Source: CAD feature listing. Evaluate the final solid. Frame: model axes, mm. A direction names the side the tool comes from. Coordinates: 2 decimals unless noted, no trailing zeros. Write each loop counter-clockwise with the first axis right and the second up, starting at its lowest first coordinate (ties: lowest second). Pieces come first, ordered by that corner, then holes. Notation, with made-up numbers: (-9.75, -9.5) - (30.25, -9.5) arc R21 ccw to (30.25, 24.5) - close; hole circle Ø1 at (-31.5, 9). An arc over 180 degrees is marked (long way). One line per item, written item: value.
from build123d import *

# Parameters (mm, degrees)
BOSS_EXTRUDE1_DEPTH       = 31
SKETCH2_W                 = 4
SKETCH2_H                 = 6
CUT_EXTRUDE1_DEPTH        = 10
CHAMFER1_SIZE             = 3
SKETCH3_R                 = 1
CUT_EXTRUDE2_DEPTH        = 12
SKETCH4_R                 = 2.75
CUT_EXTRUDE3_DEPTH        = 3
M3X0_5_TAPPED_HOLE1_D     = 2.5
M3X0_5_TAPPED_HOLE1_DEPTH = 5.5
M3X0_5_TAPPED_HOLE1_TIP   = 0.751075774
CHAMFER2_SIZE             = 1
CHAMFER3_SIZE             = 1
CHAMFER4_SIZE             = 1
CHAMFER5_SIZE             = 1
CHAMFER6_SIZE             = 1
SKETCH6_R                 = 3
CUT_EXTRUDE4_DEPTH        = 76.325976363
SKETCH7_R                 = 8.5
CUT_EXTRUDE5_DEPTH        = 8
CHAMFER7_SIZE             = 0.5
CHAMFER8_SIZE             = 0.5
SKETCH8_R                 = 3.25
CUT_EXTRUDE6_DEPTH        = 73.401676189
SKETCH9_R                 = 1
CUT_EXTRUDE7_DEPTH        = 26
CIRPATTERN1_COUNT         = 4


with BuildPart() as part:
    # Sketch1 → Boss-Extrude1 (new body)
    with BuildSketch(Plane(origin=(0, 0, 0), x_dir=(1, 0, 0), z_dir=(0, 1, 0))):
        with BuildLine():
            Line((38.438211647, 10.935520299), (38.438211647, 20.93675572))
            Line((38.438211647, 20.93675572), (42.438211647, 20.93675572))
            Line((42.438211647, 20.93675572), (42.438211647, 14.546924278))
            ThreePointArc((42.438211647, 14.546924278), (61.123879761, -10.180568437), (38.22154498, -31.06324428))
            Line((38.22154498, -31.06324428), (-18.77845502, -31.06324428))
            Line((-18.77845502, -31.06324428), (-18.77845502, 14.93675572))
            Line((-18.77845502, 14.93675572), (33.82154498, 14.93675572))
            Line((33.82154498, 14.93675572), (33.82154498, 20.93675572))
            Line((33.82154498, 20.93675572), (37.82154498, 20.93675572))
            Line((37.82154498, 20.93675572), (37.82154498, 10.932544727))
            ThreePointArc((37.82154498, 10.932544727), (38.31322372, -27.063023095), (38.438211647, 10.935520299))
        make_face()
        with BuildLine():
            Line((12, 11.93675572), (12, 1.788697084))
            Line((12, 1.788697084), (16.336864234, 1.788697084))
            ThreePointArc((16.336864234, 1.788697084), (19.928181819, 7.472291251), (24.955045819, 11.93675572))
            Line((24.955045819, 11.93675572), (12, 11.93675572))
        make_face(mode=Mode.SUBTRACT)
        with BuildLine():
            Line((12, -17.915185645), (16.336864234, -17.915185645))
            ThreePointArc((16.336864234, -17.915185645), (19.928181819, -23.598779812), (24.955045819, -28.06324428))
            Line((24.955045819, -28.06324428), (12, -28.06324428))
            Line((12, -28.06324428), (12, -17.915185645))
        make_face(mode=Mode.SUBTRACT)
    extrude(amount=BOSS_EXTRUDE1_DEPTH)

    # Sketch2 → Cut-Extrude1 (cut)
    with BuildSketch(Plane(origin=(0, 31, 0), x_dir=(1, 0, 0), z_dir=(0, 1, 0))):
        with BuildLine():
            Line((38.438211647, 20.93675572), (38.438211647, 14.93675572))
            ThreePointArc((38.438211647, 14.93675572), (40.446719395, 14.829888823), (42.438211647, 14.547962381))
            Line((42.438211647, 14.547962381), (42.438211647, 20.93675572))
            Line((42.438211647, 20.93675572), (38.438211647, 20.93675572))
        make_face()
        with Locations((35.82154498, 17.93675572)):
            Rectangle(SKETCH2_W, SKETCH2_H)
    cut_extrude1 = extrude(amount=-CUT_EXTRUDE1_DEPTH, mode=Mode.SUBTRACT)

    # Mirror1: Cut-Extrude1 across plane
    add(cut_extrude1.mirror(Plane.ZX.offset(15.5)), mode=Mode.SUBTRACT)

    # Chamfer1
    chamfer1_edges = [part.edges().sort_by_distance(p)[0] for p in [
        (40.438211647, 10, -20.93675572),
        (35.82154498, 10, -20.93675572),
        (40.438211647, 21, -20.93675572),
        (35.82154498, 21, -20.93675572),
    ]]
    chamfer(chamfer1_edges, length=CHAMFER1_SIZE)

    # Sketch3 → Cut-Extrude2 (cut)
    with BuildSketch(Plane(origin=(42.438211647, 0, 0), x_dir=(0, 0, -1), z_dir=(1, 0, 0))):
        with Locations((17.73675572, 15.5)):
            Circle(SKETCH3_R)
    extrude(amount=-CUT_EXTRUDE2_DEPTH, mode=Mode.SUBTRACT)

    # Sketch4 → Cut-Extrude3 (cut)
    with BuildSketch(Plane(origin=(42.438211647, 0, 0), x_dir=(0, 0, -1), z_dir=(1, 0, 0))):
        with Locations((17.73675572, 15.5)):
            Circle(SKETCH4_R)
    extrude(amount=-CUT_EXTRUDE3_DEPTH, mode=Mode.SUBTRACT)

    # M3x0.5 Tapped Hole1
    with Locations(Plane(origin=(33.82154498, 15.5, -17.73675572), x_dir=(0, 0, -1), z_dir=(-1, 0, 0))):
        with Locations((0, 0)):
            Hole(M3X0_5_TAPPED_HOLE1_D / 2, depth=M3X0_5_TAPPED_HOLE1_DEPTH)
            with Locations((0, 0, -(M3X0_5_TAPPED_HOLE1_DEPTH + M3X0_5_TAPPED_HOLE1_TIP / 2))):  # 118° drill point
                Cone(0, M3X0_5_TAPPED_HOLE1_D / 2, M3X0_5_TAPPED_HOLE1_TIP, mode=Mode.SUBTRACT)

    # Chamfer2
    chamfer2_edges = [part.edges().sort_by_distance(p)[0] for p in [
        (61.123879761, 31, 10.180568437),
        (9.52154498, 31, -14.93675572),
        (-18.77845502, 31, 8.06324428),
        (9.72154498, 31, 31.06324428),
    ]]
    chamfer(chamfer2_edges, length=CHAMFER2_SIZE)

    # Chamfer3
    chamfer3_edges = [part.edges().sort_by_distance(p)[0] for p in [
        (40.446719395, 31, -14.829888823),
    ]]
    chamfer(chamfer3_edges, length=CHAMFER3_SIZE)

    # Chamfer4
    chamfer4_edges = [part.edges().sort_by_distance(p)[0] for p in [
        (9.52154498, 0, -14.93675572),
        (61.123879761, 0, 10.180568437),
        (9.72154498, 0, 31.06324428),
        (-18.77845502, 0, 8.06324428),
    ]]
    chamfer(chamfer4_edges, length=CHAMFER4_SIZE)

    # Chamfer5
    chamfer5_edges = [part.edges().sort_by_distance(p)[0] for p in [
        (40.446719395, 0, -14.829888823),
    ]]
    chamfer(chamfer5_edges, length=CHAMFER5_SIZE)

    # Chamfer6
    chamfer6_edges = [part.edges().sort_by_distance(p)[0] for p in [
        (-18.77845502, 15.5, -14.93675572),
        (-18.77845502, 15.5, 31.06324428),
    ]]
    chamfer(chamfer6_edges, length=CHAMFER6_SIZE)

    # Sketch6 → Cut-Extrude4 (cut, through all)
    with BuildSketch(Plane(origin=(0, 31, 0), x_dir=(1, 0, 0), z_dir=(0, 1, 0))):
        with Locations(Location((-5.77845502, -24.06324428, 0), (0, 0, 270))):
            Circle(SKETCH6_R)
        with Locations(Location((-5.77845502, 7.93675572, 0), (0, 0, 270))):
            Circle(SKETCH6_R)
    extrude(amount=-CUT_EXTRUDE4_DEPTH, mode=Mode.SUBTRACT)

    # Sketch7 → Cut-Extrude5 (cut)
    with BuildSketch(Plane(origin=(0, 31, 0), x_dir=(1, 0, 0), z_dir=(0, 1, 0))):
        with Locations(Location((-5.77845502, -8.06324428, 0), (0, 0, 270))):
            Circle(SKETCH7_R)
    cut_extrude5 = extrude(amount=-CUT_EXTRUDE5_DEPTH, mode=Mode.SUBTRACT)

    # Chamfer7
    chamfer7_edges = [part.edges().sort_by_distance(p)[0] for p in [
        (-5.77845502, 31, -0.43675572),
    ]]
    chamfer(chamfer7_edges, length=CHAMFER7_SIZE)

    # Mirror3: Cut-Extrude5 across plane
    add(cut_extrude5.mirror(Plane.ZX.offset(15.5)), mode=Mode.SUBTRACT)

    # Chamfer8
    chamfer8_edges = [part.edges().sort_by_distance(p)[0] for p in [
        (-5.77845502, 0, -0.43675572),
    ]]
    chamfer(chamfer8_edges, length=CHAMFER8_SIZE)

    # Sketch8 → Cut-Extrude6 (cut, through all)
    with BuildSketch(Plane(origin=(0, 23, 0), x_dir=(1, 0, 0), z_dir=(0, 1, 0))):
        with Locations(Location((-5.77845502, -8.06324428, 0), (0, 0, 270))):
            Circle(SKETCH8_R)
    extrude(amount=-CUT_EXTRUDE6_DEPTH, mode=Mode.SUBTRACT)

    # Sketch9 → Cut-Extrude7 (cut)
    with BuildSketch(Plane(origin=(0, 23, 0), x_dir=(1, 0, 0), z_dir=(0, 1, 0))):
        with Locations(Location((-5.77845502, -1.86324428, 0), (0, 0, 270))):
            Circle(SKETCH9_R)
    cut_extrude7 = extrude(amount=-CUT_EXTRUDE7_DEPTH, mode=Mode.SUBTRACT)

    # Sketch10 → M3x0.5 Tapped Hole2 (revolve, cut)
    with BuildSketch(Plane(origin=(-5.77845502, 23, 1.86324428), x_dir=(0, 0, 1), z_dir=(1, 0, 0))):
        Polygon((0, 0), (0, 27.251075774), (1.25, 26.5), (1.25, 0), align=None)
    m3x0_5_tapped_hole2 = revolve(axis=Axis((-5.77845502, 29.35, 1.86324428), (0, -1, 0)), mode=Mode.SUBTRACT)

    # CirPattern1: Cut-Extrude7, M3x0.5 Tapped Hole2 ×4 about axis
    cirpattern1_axis = Axis((-5.77845502, 0, 8.06324428), (0, 1, 0))
    add([cut_extrude7.rotate(cirpattern1_axis, i * 360 / CIRPATTERN1_COUNT) for i in range(1, CIRPATTERN1_COUNT)], mode=Mode.SUBTRACT)
    add([m3x0_5_tapped_hole2.rotate(cirpattern1_axis, i * 360 / CIRPATTERN1_COUNT) for i in range(1, CIRPATTERN1_COUNT)], mode=Mode.SUBTRACT)


solid = part.part
1) Material intervals for line 1 (Z direction, x = -5.5, y = 6.5); line 2 (Z direction, x = 38.75, y = 15.5); line 3 (X direction, y = 17.5, z = 23), sorted ascending.
Values found:
line 1: -14.94 to -10.92, -4.95 to -0.43, 16.56 to 21.08, 27.05 to 31.06
line 2: -20.94 to -18.99, -16.49 to -10.93, 27.06 to 31.06
line 3: -18.78 to -8.58, -2.97 to 12, 19.44 to 26.48, 49.96 to 55.71
2) Draft query along X for faces 6 (the conical face through (60.339, 30.826, 9.647)), 7 (the flat face through (35.794, 19.521, -19.416)), 8 (the cylindrical face through (-10.786, 15.605, 8.439)). Return one class per face: released by +X, released by -X, zero draft, split by the parting line, or undercut.
Values found:
face 6: released by +X
face 7: zero draft
face 8: undercut
3) Contact query for flat-ended pins moving along their axis: P1, Ø7, axis at y = 15.5, z = -17.74, coming from the -X side; P2, Ø5, axis at x = -5.78, z = 24.06, coming from the +Y side; P3, Ø11, axis at y = 12, z = 24.5, coming from the +X side; P4, Ø1.7, axis at x = 41, z = -16, coming from the +Y side. Output: stop coordinate, or through.
Values found:
P1: x = -18.48
P2: through
P3: x = 58.45
P4: y = 21
4) Section query B-B on x = 29. Output: boundary loops of the cut face in (y, z).
Values found:
outline: (0, -13.94) - (1, -14.94) - (30, -14.94) - (31, -13.94) - (31, -8.55) - (0, -8.55) - close; (0, 24.68) - (31, 24.68) - (31, 30.06) - (30, 31.06) - (1, 31.06) - (0, 30.06) - close
5) Section query A-A on y = 28.5. State how many separate pieces and enclosed holes the cut face has, then the cut area to 3 significant figures.
Values found:
separate pieces: 1
enclosed holes: 5
area: 1,870 mm2
6) Reachability of faces 1 (the flat face through (33.822, 17, -17)), 2 (the cylindrical face through (-13.319, 4.198, 11.985)), 3 (the cylindrical face through (38.89, 14.26, -17.9)), 4 (the flat face through (12, 15, -7)), 5 (the flat face through (36, 21, -16)) from +Z, -Z, +X, -X, +Y, -Y: full face, straight path, thin tool, end or side. Return the list, or none.
Values found:
face 1: -Z, -X, +Y, -Y
face 2: -Y
face 3: -X
face 4: +Y, -Y
face 5: -Z, +X, -X, +Y
